Source: CAD feature listing. Evaluate the final solid. Frame: model axes, mm. A direction names the side the tool comes from. Give positions to 0.01 mm unless a question says otherwise; leave off trailing zeros. Order: outer loops, then holes, each group sorted by start corner. A loop starts at its lowest first (then second) coordinate and runs counter-clockwise, first axis right, second up. Notation, with made-up numbers: (36, 11.5) - (86, 11.5) arc R22 cw to (86, 47.5) - close; hole circle Ø5 at (58.25, -35.75). An arc over 180 degrees is marked (long way). Answer as CSV lines item,"result".
```python
from build123d import *

# Parameters (mm, degrees)
CUT_EXTRUDE1_START = 38.1
SKETCH4_W          = 12.7
SKETCH4_H          = 9.906
CUT_EXTRUDE1_DEPTH = 15.24


with BuildPart() as part:
    # Sketch2 → Revolve2 (revolve)
    with BuildSketch(Plane(origin=(0, 0, 0), x_dir=(0, 0, -1), z_dir=(1, 0, 0)), mode=Mode.PRIVATE) as revolve2_sk:
        Polygon((0, 0), (0, 6.35), (38.1, 44.45), (44.45, 44.45), (44.45, 38.1), (6.35, 0), align=None)
    revolve(revolve2_sk.sketch.rotate(Axis((0, 0, -6.35), (0, 0, 1)), 90), axis=Axis((0, 0, -6.35), (0, 0, 1)))

    # Sketch4 → Cut-Extrude1 (cut)
    with BuildSketch(Plane(origin=(0, 0, 0), x_dir=(1, 0, 0), z_dir=(0, 1, 0)).offset(CUT_EXTRUDE1_START)):
        with Locations((0, 23.373056835)):
            Rectangle(SKETCH4_W, SKETCH4_H)
    extrude(amount=-CUT_EXTRUDE1_DEPTH, mode=Mode.SUBTRACT)


solid = part.part
```
(1) Contact query for flat-ended pins moving along their axis: pin 1 (12 mm diameter, centred on x = 34, y = -22.5, fed in from +Z); pin 2 (1 mm diameter, centred on x = 19.5, y = 3.5, fed in from +Z); pin 3 (4 mm diameter, centred on y = 8.5, z = -15, fed in from +X). Output: stop coordinate, or through.
Completed:
pin 1,"z = -28.42"
pin 2,"z = -12.96"
pin 3,"x = 21.88"
(2) Cut plane B-B (z = -34). Return loops of the section in (x, y), then the cut area to 3 significant figures.
Completed:
outline,"circle Ø80.7 at (0, 0); hole circle Ø55.3 at (0, 0)"
area,"2,710 mm²"
(3) Access query for faces 1 (the flat face through (-6.35, 27, -24)), 2 (the flat face through (0, 0, 0)). Directions: +Z, -Z, +X, -X, +Y, -Y. A direction counts if a zero-diameter tool reaches every point of the face in a straight line with its end or side. Return the directions, or none.
Completed:
face 1,"+Y"
face 2,"+Z, +X, -X, +Y, -Y"
(4) Cut plane A-A (z = -41). Return loops of the section in (x, y), then the cut area to 3 significant figures.
Completed:
outline,"circle Ø88.9 at (0, 0); hole circle Ø69.3 at (0, 0)"
area,"2,440 mm²"
(5) Mould query, pull axis Z, two halves, no side actions, for faces 3 (the flat face through (6.35, 27, -24)), 4 (the conical face through (-6.971, -10.934, -6.617)), 5 (the conical face through (8.19, 6.28, -16.67)). Classes: released by +Z, released by -Z, zero draft, split by the parting line, or undercut.
Completed:
face 3,"undercut"
face 4,"released by +Z"
face 5,"released by -Z"
(6) Ray query, line 1 (Y direction, x = 1.5, z = -39); line 2 (Y direction, x = -5, z = -22.5); line 3 (Y direction, x = 11, z = -7.5). Return the intervals inside material, ascending. Write a range as from..to.
Completed:
line 1,"-44.42..-32.62, 32.62..44.42"
line 2,"-28.41..-15.36, 15.36..22.86"
line 3,"-8.42..8.42"
